Geometry: final body of the model. Coordinates: model frame, mm. A direction names the side the tool comes from. Coordinates: 2 decimals unless noted, no trailing zeros. Loops run counter-clockwise (first coordinate to the right, second up) from the corner with the lowest first, then second, coordinate; pieces in that order, holes last. Notation, with made-up numbers: (-17, 16) - (15, 16) arc R14 ccw to (15, 38) - close; hole circle Ø2 at (-21.75, 22.25). An arc over 180 degrees is marked (long way). Put each result on its own line as item: value. Start each with the question number.
1) Material intervals for line 1 along Z through (x, y) = (25, 71.25); line 2 along Z through (x, y) = (-12.5, 68.2); line 3 along X through (y, z) = (72.75, -30.75), sorted ascending. Write a range as from..to.
2) Reachability of faces 1 (the flat face through (-8, 72, -33)), 2 (the flat face through (20, 69, -23)), 3 (the flat face through (0, 70, -30)) from +Z, -Z, +X, -X, +Y, -Y: full face, straight path, thin tool, end or side. Return the list, or none.
3) Section C-C on y = 68.25. Output: boundary loops of the cut face in (x, z).
4) Section B-B on x = 0. Output: boundary loops of the cut face in (y, z).
5) Section D-D on z = -18. Output: boundary loops of the cut face in (x, y), and give its area (3 significant figures).
6) Draft query along Z for faces 4 (the flat face through (25, 72, -15)), 5 (the cylindrical face through (0, 70, -20)), 6 (the flat face through (0, 67, -19)). Return one class per face: +Z half, -Z half, draft (parallel to the pull), parting line (faces both ways), or undercut.
7) Contact query for flat-ended pins moving along their axis: pin 1 Ø4 at (x, y) = (-6, 71) entering from -Z; pin 2 Ø3 at (x, z) = (-12.5, -22.5) entering from -Y; pin 3 Ø6 at (x, z) = (-25, -22.5) entering from +Y. Output: stop coordinate, or through.
8) Section A-A on z = -22.5. Count the separate pieces of the cut face and the enclosed holes in it, and give its area (3 significant figures).
```python
from build123d import *

# Parameters (mm, degrees)
PAD017_DEPTH        = 5
HOLE001_D           = 3.6
HOLE001_DEPTH       = 25
HOLE001_CSINK_D     = 7.5
HOLE001_CSINK_ANGLE = 90
SKETCH026_W         = 40
SKETCH026_H         = 15
PAD018_DEPTH        = 3
SKETCH027_R         = 2.5
POCKET006_DEPTH     = 5


with BuildPart() as part:
    # Sketch024 → Pad017 (new body)
    with BuildSketch(Plane.XZ.offset(-70)):
        Polygon((-30, -20), (-30, -35), (-10, -35), (-5, -30), (5, -30), (10, -35), (30, -35), (30, -20), (20, -10), (-20, -10), align=None)
    extrude(amount=-PAD017_DEPTH)

    # Hole001
    with Locations(Plane(origin=(0, 75, 0), x_dir=(1, 0, 0), z_dir=(0, 1, 0))):
        with Locations((25, 22.5), (25, 30), (-25, 30), (-25, 22.5)):
            CounterSinkHole(HOLE001_D / 2, HOLE001_CSINK_D / 2, depth=HOLE001_DEPTH, counter_sink_angle=HOLE001_CSINK_ANGLE)

    # Sketch026 → Pad018 (join)
    with BuildSketch(Plane.XZ.offset(-70)):
        with Locations((0, -22.5)):
            Rectangle(SKETCH026_W, SKETCH026_H)
    extrude(amount=PAD018_DEPTH)

    # Sketch027 → Pocket006 (cut)
    with BuildSketch(Plane.XZ.offset(-72)):
        with Locations((-12.5, -22.5)):
            Circle(SKETCH027_R)
        with Locations((0, -22.5)):
            Circle(SKETCH027_R)
        with Locations((12.5, -22.5)):
            Circle(SKETCH027_R)
    extrude(amount=POCKET006_DEPTH, mode=Mode.SUBTRACT)


solid = part.part
```
Answer block:
1. line 1: z = -35..-31.8, -28.2..-24.3, -20.7..-15
1. line 2: z = -30..-25, -20..-15
1. line 3: x = -30..-26.64, -23.36..-5.75, 5.75..23.36, 26.64..30
2. face 1: -Z, +Y, -Y
2. face 2: +Z, -Z, +X, -Y
2. face 3: -Z, -Y
3. outline: (-20, -30) - (20, -30) - (20, -15) - (-20, -15) - close; hole circle Ø5 at (-12.5, -22.5); hole circle Ø5 at (0, -22.5); hole circle Ø5 at (12.5, -22.5)
4. outline: (67, -30) - (75, -30) - (75, -10) - (70, -10) - (70, -15) - (67, -15) - (67, -20) - (72, -20) - (72, -25) - (67, -25) - close
5. outline: (-28, 70) - (-20, 70) - (-20, 67) - (20, 67) - (20, 70) - (28, 70) - (28, 75) - (-28, 75) - close
5. area: 400 mm²
6. face 4: +Z half
6. face 5: undercut
6. face 6: draft
7. pin 1: stops at z = -33
7. pin 2: stops at y = 72
7. pin 3: stops at y = 74.25
8. separate pieces: 3
8. enclosed holes: 0
8. area: 301 mm²
